Model file for the job. Use its own axes, mm. Face numbers are marked on the shaded views. A direction names the side the tool comes from. Round coordinates to 2 decimals unless told otherwise and drop trailing zeros. Loops run counter-clockwise (first coordinate to the right, second up) from the corner with the lowest first, then second, coordinate; pieces in that order, holes last. Notation, with made-up numbers: (-34, 26) -> (17, 26) arc R24 cw to (17, 37) -> close; hole circle Ø3 at (27, 67.5). An arc over 180 degrees is marked (long way). Use a Markdown table: item, result. Add a question column.
```python
from build123d import *

# Parameters (mm, degrees)
F0_W          = 65
F0_H          = 18
F1_DEPTH      = 35
F3_DEPTH      = 70.001
F4_R          = 2
F5_R          = 1
F6_W          = 7
F6_H          = 3
F7_DEPTH      = 7.5
F8_W          = 58
F8_H          = 50
F9_DEPTH      = 7
F10_T1_DEPTH  = 50
F10_T3_DEPTH  = 58
F10_T8_DEPTH  = 65.7150489639
F10_T13_DEPTH = 58
F10_T18_DEPTH = 65.7150489639


# Not quite as in the source:
# - a fillet or chamfer that OpenCascade refuses, or shapes differently, is made with other operations: its cross-section is extruded or revolved along the edge and cut away or added


with BuildPart() as f1:
    # F0 (on Right) → F1 (new body, symmetric)
    with BuildSketch(Plane.YZ):
        Rectangle(F0_W, F0_H)
    extrude(amount=F1_DEPTH, both=True)

    # F2 (on face) → F3 (cut, through all)
    with BuildSketch(Plane.YZ.offset(35)):
        Polygon((-14.8550952894, 9), (-27.5, 9), (-26.1775476447, 1.5), (-16.1775476447, 1.5), align=None)
        Polygon((-21.5490479022, 13.5265095159), (-32.5, 9), (-27.5, 9), (-14.8550952894, 9), align=None)
    extrude(amount=-F3_DEPTH, mode=Mode.SUBTRACT)

    # F4
    f4_edges = [f1.edges().sort_by_distance(p)[0] for p in [
        (0, -14.855095, 9),
        (0, -27.5, 9),
    ]]
    fillet(f4_edges, radius=F4_R)

    # F5
    f5_edges = [f1.edges().sort_by_distance(p)[0] for p in [
        (35, 9.661552, 9),
        (35, -30.8391, 9),
        (35, -27.892624, 8.532089),
        (35, -32.5, 0),
        (35, -26.693066, 4.423648),
        (35, 0, -9),
        (35, -21.177548, 1.5),
        (35, 32.5, 0),
        (35, -15.66203, 4.423648),
        (35, -14.462471, 8.532089),
        (-35, 32.5, 0),
        (0, 32.5, 9),
        (0, 32.5, -9),
        (-35, -30.8391, 9),
        (-35, -27.892624, 8.532089),
        (-35, -32.5, 0),
        (-35, -26.693066, 4.423648),
        (-35, 0, -9),
        (-35, -21.177548, 1.5),
        (-35, -15.66203, 4.423648),
        (-35, 9.661552, 9),
        (-35, -14.462471, 8.532089),
    ]]
    fillet(f5_edges, radius=F5_R)

    # F6 (on Right) → F7 (cut, symmetric)
    with BuildSketch(Plane.YZ):
        with Locations((-21.1775476447, -1)):
            Rectangle(F6_W, F6_H)
        with Locations((-21.1775476447, 2)):
            Rectangle(F6_W, F6_H)
    extrude(amount=F7_DEPTH, both=True, mode=Mode.SUBTRACT)

    # F8 (on face) → F9 (cut)
    with BuildSketch(Plane(origin=(0, 0, -9), x_dir=(1, 0, 0), z_dir=(0, 0, -1))):
        Rectangle(F8_W, F8_H)
    extrude(amount=-F9_DEPTH, mode=Mode.SUBTRACT)

    # F10: chamfer of 3 on 4 edges, made by hand

    # F10_s2 → F10_t1 (join)
    with BuildSketch(Plane.XZ.offset(-25)):
        Polygon((26, -2), (29, -5), (29, -2), align=None)
        Polygon((-26, -2), (-29, -5), (-29, -2), align=None)
    extrude(amount=F10_T1_DEPTH)

    # F10_s4 → F10_t3 (join)
    with BuildSketch(Plane.YZ.offset(-29)):
        Polygon((22, -2), (25, -5), (25, -2), align=None)
    extrude(amount=F10_T3_DEPTH)


with BuildPart() as f10_tool6:
    # F10_s7 → F10_t8 (new body)
    with BuildSketch(Plane.YZ.offset(29)):
        Polygon((-22, -2), (-25, -5), (-25, -2), align=None)
    extrude(amount=-F10_T8_DEPTH)

    split(bisect_by=Plane.YZ.offset(7.5), keep=Keep.TOP)


with BuildPart() as f1_1:
    add(f1.part)

    # F10_t5: union F10_tool6
    add(f10_tool6.part)


with BuildPart() as f10_tool11:
    # F10_s12 → F10_t13 (new body)
    with BuildSketch(Plane.YZ.offset(29)):
        Polygon((-22, -2), (-25, -5), (-25, -2), align=None)
    extrude(amount=-F10_T13_DEPTH)

    split(bisect_by=Plane.XZ.offset(24.6775476447), keep=Keep.TOP)


with BuildPart() as f1_2:
    add(f1_1.part)

    # F10_t10: union F10_tool11
    add(f10_tool11.part)


with BuildPart() as f10_tool16:
    # F10_s17 → F10_t18 (new body)
    with BuildSketch(Plane.YZ.offset(36.7150489639)):
        Polygon((-22, -2), (-25, -5), (-25, -2), align=None)
    extrude(amount=-F10_T18_DEPTH)

    split(bisect_by=Plane.YZ.offset(-7.5), keep=Keep.BOTTOM)


with BuildPart() as f1_3:
    add(f1_2.part)

    # F10_t15: union F10_tool16
    add(f10_tool16.part)


solid = f1_3.part
```
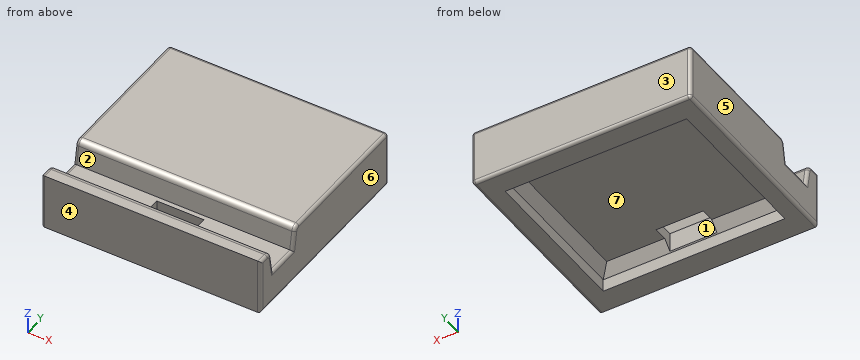
1) Cut at B-B on z = -0.5. Write the cut outline in (x, y), and give its area (3 significant figures).
2) Cut at C-C on y = 9. Write the cut outline in (x, z), and give its area (3 significant figures).
3) Cut at D-D on x = -24. Write the cut outline in (y, z).
4) Wall check: probe 1 along X at (y, z) = (12.5, -7.25); probe 2 along Y at (x, z) = (-9, -5); probe 3 along Z at (x, y) = (19.5, -11). Give the ranges that are in metal, low to high. Write a range as from..to.
5) Pin check, flat tips, straight feed: pin 1 Ø5 at (x, y) = (-16.5, -22.5) entering from +Z; pin 2 Ø10 at (x, y) = (2, -7.5) entering from -Z. Stop position of each tip, or through.
6) Tool access for the marked faces 1, 2 and 3: list every direction of +Z, -Z, +X, -X, +Y, -Y with a clear straight run to the whole face (end or side of a thin tool).
7) Cut at A-A on x = 0. Write the cut outline in (y, z).
8) Pull direction X, two halves, no side cores. Call the marked faces 4, 5, 6 and 7: +X half, -X half, draft (parallel to the pull), parting line (faces both ways), or undercut.
Established:
| question | item | result |
|---|---|---|
| 1 | outline | (-35, -31.5) arc R1 ccw to (-34, -32.5) -> (34, -32.5) arc R1 ccw to (35, -31.5) -> (35, 31.5) arc R1 ccw to (34, 32.5) -> (-34, 32.5) arc R1 ccw to (-35, 31.5) -> close; hole (-7.5, -24.68) -> (7.5, -24.68) -> (7.5, -17.68) -> (-7.5, -17.68) -> close |
| 1 | area | 4,440 mm^2 |
| 2 | outline | (-35, -8) arc R1 ccw to (-34, -9) -> (-29, -9) -> (-29, -5) -> (-26, -2) -> (26, -2) -> (29, -5) -> (29, -9) -> (34, -9) arc R1 ccw to (35, -8) -> (35, 8) arc R1 ccw to (34, 9) -> (-34, 9) arc R1 ccw to (-35, 8) -> close |
| 2 | area | 862 mm^2 |
| 3 | outline | (-32.5, -9) -> (-25, -9) -> (-25, -5) -> (-22, -2) -> (22, -2) -> (25, -5) -> (25, -9) -> (31.5, -9) arc R1 ccw to (32.5, -8) -> (32.5, 8) arc R1 ccw to (31.5, 9) -> (-13.18, 9) arc R2 ccw to (-15.15, 7.35) -> (-16.18, 1.5) -> (-26.18, 1.5) -> (-27.21, 7.35) arc R2 ccw to (-29.18, 9) -> (-32.5, 9) -> close |
| 4 | probe 1 | x = -35..-29, 29..35 |
| 4 | probe 2 | y = -32.5..-25, 25..32.5 |
| 4 | probe 3 | z = -2..9 |
| 5 | pin 1 | stops at z = 1.5 |
| 5 | pin 2 | stops at z = -2 |
| 6 | face 1 | +Z, -Z |
| 6 | face 2 | +Z, +X, -X |
| 6 | face 3 | +Z, -Z, +X, -X, +Y |
| 7 | outline | (-32.5, -9) -> (-25, -9) -> (-25, -5) -> (-24.68, -4.68) -> (-24.68, 1.5) -> (-26.18, 1.5) -> (-27.21, 7.35) arc R2 ccw to (-29.18, 9) -> (-32.5, 9) -> close; (-17.68, -2) -> (22, -2) -> (25, -5) -> (25, -9) -> (31.5, -9) arc R1 ccw to (32.5, -8) -> (32.5, 8) arc R1 ccw to (31.5, 9) -> (-13.18, 9) arc R2 ccw to (-15.15, 7.35) -> (-16.18, 1.5) -> (-17.68, 1.5) -> close |
| 8 | face 4 | draft |
| 8 | face 5 | -X half |
| 8 | face 6 | +X half |
| 8 | face 7 | undercut |
